Here's how the part is built. I have some questions about the finished solid (model axes, mm). A direction names the side the tool comes from. Round coordinates to 2 decimals unless told otherwise and drop trailing zeros. Loops run counter-clockwise (first coordinate to the right, second up) from the corner with the lowest first, then second, coordinate; pieces in that order, holes last. Notation, with made-up numbers: M 50.25,8.25 L 77.25,8.25 A14 ccw 77.25,13.25 Z; hole C -30,1.5 d4. An arc over 180 degrees is marked long. Use a Markdown table: item, result.
from build123d import *

# Parameters (mm, degrees)
SKETCH_R        = 31.9
SKETCH_R_2      = 6
PAD_DEPTH       = 2
SKETCH001_R     = 31.9
SKETCH001_R_2   = 30
PAD001_DEPTH    = 2
PAD002_DEPTH    = 2
CHAMFER_SIZE    = 1
CHAMFER001_SIZE = 0.3


with BuildPart() as part:
    # Sketch → Pad (new body)
    with BuildSketch(Plane.XY):
        Circle(SKETCH_R)
        with Locations((9.999037, 20.71278)):
            Circle(SKETCH_R_2, mode=Mode.SUBTRACT)
        with Locations((22.937312, 1.69697)):
            Circle(SKETCH_R_2, mode=Mode.SUBTRACT)
        with Locations((12.938275, -19.01581)):
            Circle(SKETCH_R_2, mode=Mode.SUBTRACT)
        with Locations((-9.999037, -20.71278)):
            Circle(SKETCH_R_2, mode=Mode.SUBTRACT)
        with Locations((-22.937312, -1.69697)):
            Circle(SKETCH_R_2, mode=Mode.SUBTRACT)
        with Locations((-12.938275, 19.01581)):
            Circle(SKETCH_R_2, mode=Mode.SUBTRACT)
        Polygon((0, 16.627688), (-14.4, 8.313844), (-14.4, -8.313844), (0, -16.627688), (14.4, -8.313844), (14.4, 8.313844), align=None, mode=Mode.SUBTRACT)
    extrude(amount=PAD_DEPTH)

    # Sketch001 (on Face15 of Pad) → Pad001 (join)
    with BuildSketch(Plane.XY.offset(2)):
        Circle(SKETCH001_R)
        Circle(SKETCH001_R_2, mode=Mode.SUBTRACT)
    extrude(amount=PAD001_DEPTH)

    # Sketch002 (on Face17 of Pad001) → Pad002 (join)
    with BuildSketch(Plane.XY.offset(2)):
        Polygon((0, 19.052559), (-16.5, 9.526279), (-16.5, -9.526279), (0, -19.052559), (16.5, -9.526279), (16.5, 9.526279), align=None)
        Polygon((0, 16.627688), (-14.4, 8.313844), (-14.4, -8.313844), (0, -16.627688), (14.4, -8.313844), (14.4, 8.313844), align=None, mode=Mode.SUBTRACT)
    extrude(amount=PAD002_DEPTH)

    # Chamfer
    chamfer_edges = [part.edges().sort_by_distance(p)[0] for p in [
        (-31.9, 0, 0),
    ]]
    chamfer(chamfer_edges, length=CHAMFER_SIZE)

    # Chamfer001
    chamfer001_edges = [part.edges().sort_by_distance(p)[0] for p in [
        (-7.2, -12.470766, 4),
        (-14.4, 0, 4),
        (-7.2, 12.470766, 4),
        (7.2, 12.470766, 4),
        (14.4, 0, 4),
        (7.2, -12.470766, 4),
    ]]
    chamfer(chamfer001_edges, length=CHAMFER001_SIZE)


solid = part.part
1. For pin 1 Ø7 at (x, y) = (12.94, -19.02) entering from -Z; pin 2 Ø1.8 at (y, z) = (3.5, 2) entering from +X; pin 3 Ø1.6 at (y, z) = (1.5, 2.5) entering from +X; pin 4 Ø1.6 at (y, z) = (-2, 3.5) entering from -X, each with a flat end and sliding along its axis, tell me the tip position at first contact or that it passes through.
Answer sheet:
| item | result |
|---|---|
| pin 1 | through |
| pin 2 | x = 31.79 |
| pin 3 | x = 31.89 |
| pin 4 | x = -31.88 |
2. Imagine slicing it at A-A, the plane y = 0. Write out the boundary of the cut face in (x, z).
Answer sheet:
| item | result |
|---|---|
| outline | M -31.9,1 L -30.9,0 L -28.69,0 L -28.69,2 L -30,2 L -30,4 L -31.9,4 Z; M -17.18,0 L -14.4,0 L -14.4,3.7 L -14.7,4 L -16.5,4 L -16.5,2 L -17.18,2 Z; M 14.4,0 L 17.18,0 L 17.18,2 L 16.5,2 L 16.5,4 L 14.7,4 L 14.4,3.7 Z; M 28.69,0 L 30.9,0 L 31.9,1 L 31.9,4 L 30,4 L 30,2 L 28.69,2 Z |
3. We'd pull the mould along Y, two halves only. Please class faces 4 (the face through (-7.17, 12.66, 3.85)), 5 (the face through (30.427, 9.582, 2.479)), 6 (the face through (12, -28, 4)): +Y half, -Y half, draft (parallel to the pull), parting line (faces both ways), or undercut.
Answer sheet:
| item | result |
|---|---|
| face 4 | undercut |
| face 5 | parting line |
| face 6 | draft |
4. Which directions (+Z, -Z, +X, -X, +Y, -Y) give clear straight access to the entire face, cutting with the end or side of a thin tool? Please do faces 1 (the face through (-15, 0, 4)), 2 (the face through (7.17, -12.66, 3.85)), 3 (the face through (14.4, 0, 2)).
Answer sheet:
| item | result |
|---|---|
| face 1 | +Z, +X, -X, +Y, -Y |
| face 2 | +Z |
| face 3 | +Z, -Z |
5. Imagine slicing it at B-B, the plane x = -9. State how many separate pieces and enclosed holes the cut face has, then the cut area to 3 significant figures.
Answer sheet:
| item | result |
|---|---|
| separate pieces | 4 |
| enclosed holes | 0 |
| area | 51.4 mm2 |
6. I need wall thicknesses on probe 1 along Y at (x, z) = (-12, 2.7); probe 2 along X at (y, z) = (-3.5, 1.8); probe 3 along X at (y, z) = (-23, 1.4). Which ranges of each line are inside material? Lowest first, please. Write a range as from..to.
Answer sheet:
| item | result |
|---|---|
| probe 1 | -29.56..-27.5, -12.12..-9.7, 9.7..12.12, 27.5..29.56 |
| probe 2 | -31.71..-28.66, -17.21..-14.4, 14.4..19.94, 25.94..31.71 |
| probe 3 | -22.1..-15.55, -4.45..8.45, 17.42..22.1 |
